Verification items for this drawing (mm, ordinates from the low corner). Round coordinates to 2 decimals unless told otherwise and drop trailing zeros. Order: outer loops, then holes, each group sorted by start corner. A loop starts at its lowest first (then second) coordinate and runs counter-clockwise, first axis right, second up. Notation, with made-up numbers: (39.25, -26.5) - (84.25, -26.5) arc R13 cw to (84.25, -10.5) - close; hole circle Ø2 at (36.5, 38). An arc over 180 degrees is marked (long way). Use a Markdown table: item, result. Add a question column.
(1) Section check D-D on z = 11. Record the boundary of the cut face in (x, y), then the cut area to 3 significant figures.
(2) Section check B-B on y = 7.75. Record the boundary of the cut face in (x, z), then the cut area to 3 significant figures.
(3) Section check C-C on x = 17. Record the boundary of the cut face in (y, z), then the cut area to 3 significant figures.
(4) Thickness scan on line 1 along Z through (x, y) = (14.5, 9.25) (1 decimal); line 2 along Z through (x, y) = (20, 2); line 3 along X through (y, z) = (9.5, 9). Record the ranges inside material, lowest first. Write a range as [from, to].
(5) Mould release check, pull along X, two halves, no side actions. Record for the marked faces 1, 2 and 3: released by +X, released by -X, zero draft, split by the parting line, or undercut.
(6) Section check A-A on z = 7.25. Record the boundary of the cut face in (x, y).
(7) Gauge pin test, flat ends, axial feed: P1, Ø4, axis at y = 4.5, z = 8.5, coming from the +X side; P2, Ø1.5, axis at y = 1, z = 16, coming from the -X side (1 decimal); P3, Ø2, axis at y = 4, z = 10.5, coming from the -X side; P4, Ø2, axis at x = 11.5, z = 16, coming from the +Y side. Record the tip position at first contact, or that the pin passes through.
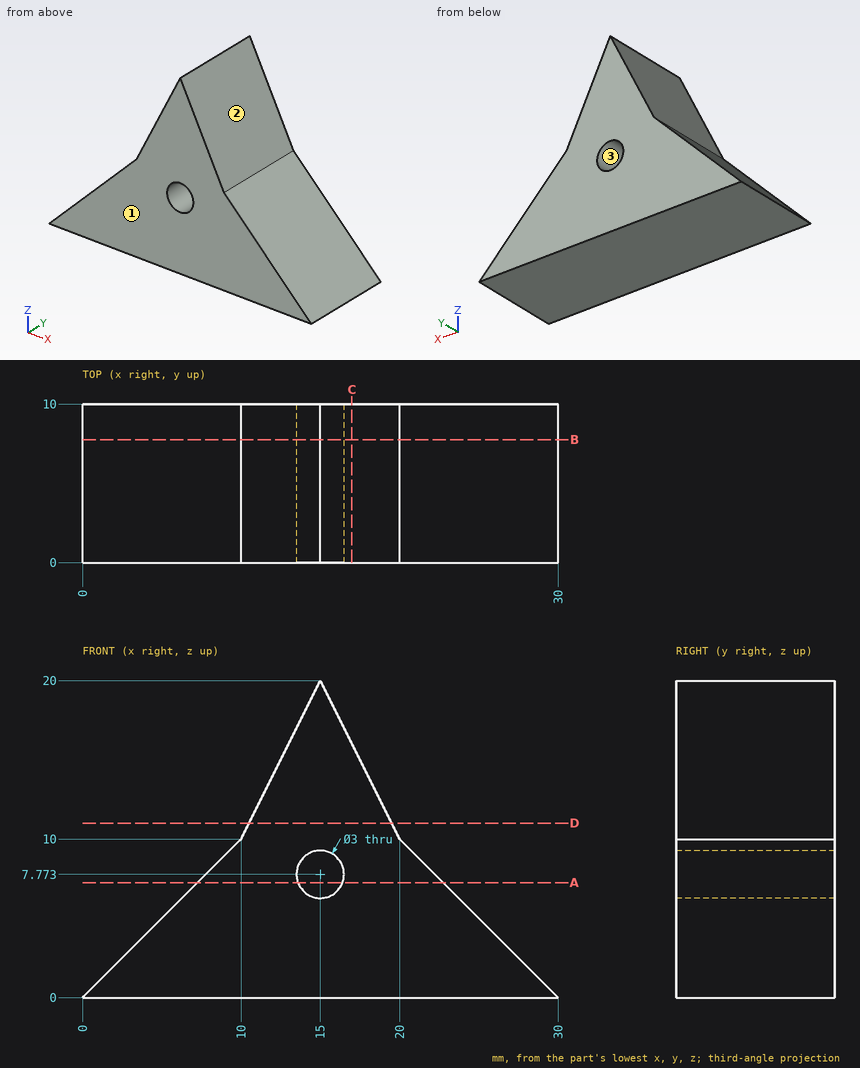
Check sheet entries:
| question | item | result |
|---|---|---|
| 1 | outline | (10.5, 0) - (19.5, 0) - (19.5, 10) - (10.5, 10) - close |
| 1 | area | 90.0 mm2 |
| 2 | outline | (0, 0) - (30, 0) - (20, 10) - (15, 20) - (10, 10) - close; hole circle Ø3 at (15, 7.77) |
| 2 | area | 243 mm2 |
| 3 | outline | (0, 0) - (10, 0) - (10, 16) - (0, 16) - close |
| 3 | area | 160 mm2 |
| 4 | line 1 | z = [0, 6.4], [9.2, 19] |
| 4 | line 2 | z = [0, 10] |
| 4 | line 3 | x = [9, 14.14], [15.86, 21] |
| 5 | face 1 | zero draft |
| 5 | face 2 | released by +X |
| 5 | face 3 | undercut |
| 6 | outline | (7.25, 0) - (13.59, 0) - (13.59, 10) - (7.25, 10) - close; (16.41, 0) - (22.75, 0) - (22.75, 10) - (16.41, 10) - close |
| 7 | P1 | stops at x = 23.5 |
| 7 | P2 | stops at x = 12.6 |
| 7 | P3 | stops at x = 9.5 |
| 7 | P4 | passes through |
